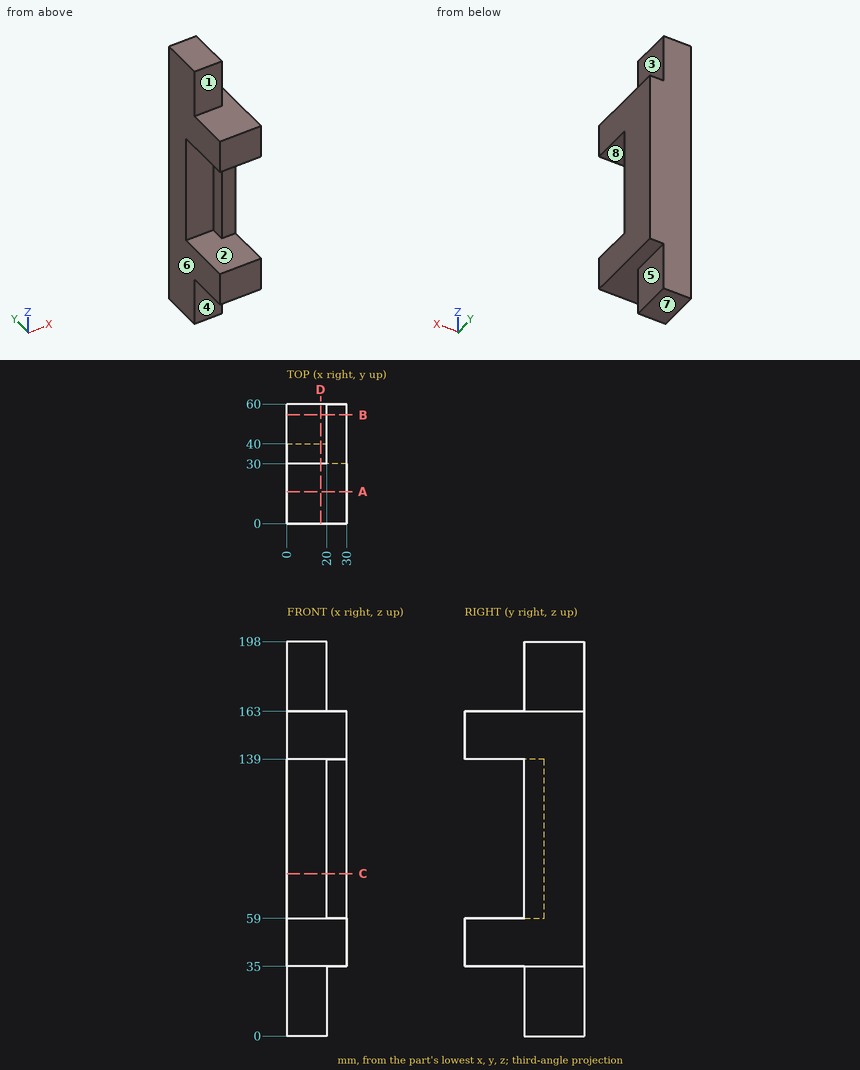
Can you work these out from the drawing? Everything is in mm from the part's minimum corner. A direction names the side the tool comes from. Give positions to 0.01 mm unless a question says otherwise; leave off trailing zeros. Write each loop counter-clockwise with the first axis right and the second up, starting at its lowest first coordinate (ties: lowest second). Pieces come first, ordered by that corner, then holes. Notation, with made-up numbers: M 40,3.5 L 46,3.5 A32 ccw 46,41.5 Z; hole C 76,-2 d2. An arc over 180 degrees is marked long. Answer in a Markdown table with one row per item. Add a question column.
Item 1: Imagine slicing it at D-D, the plane x = 17. Write out the boundary of the cut face in (y, z), plus the area to 3 significant figures.
Item 2: On a 3-axis mill with a long thin cutter (end or side, diameter ignored), from which of +Z, -Z, +X, -X, +Y, -Y can I reach the whole of each face in a straight line? I mean the marked faces 1, 2, 3, 4 and 5. Say none if no direction works.
Item 3: We'd pull the mould along Z, two halves only. Please class the marked faces 6, 7 and 8: released by +Z, released by -Z, zero draft, split by the parting line, or undercut.
Item 4: Imagine slicing it at A-A, the plane y = 16. Write out the boundary of the cut face in (x, z).
Item 5: Please list where these lines run through material, in increasing order: L1, parallel to Z at x = 11, y = 10.5; L2, parallel to Z at x = 4, y = 38; L3, parallel to Y at x = 25.25, z = 96.
Item 6: Imagine slicing it at C-C, the plane z = 81.5. Write out the boundary of the cut face in (x, y), plus the area to 3 significant figures.
Item 7: Imagine slicing it at B-B, the plane y = 54.5. Write out the boundary of the cut face in (x, z), plus the area to 3 significant figures.
Item 8: For pin 1 Ø6 at (x, z) = (13.5, 25) entering from -Y; pin 2 Ø15 at (x, y) = (10, 37.5) entering from -Z; pin 3 Ø10 at (x, y) = (6.5, 24) entering from +Z; pin 4 Ø24 at (y, z) = (43, 179) entering from +X, each with a flat end and sliding along its axis, tell me the tip position at first contact or that it passes through.
Evaluation:
| question | item | result |
|---|---|---|
| 1 | outline | M 0,35 L 30,35 L 30,0 L 60,0 L 60,198 L 30,198 L 30,163 L 0,163 L 0,139 L 40,139 L 40,59 L 0,59 Z |
| 1 | area | 6,580 mm² |
| 2 | face 1 | +Z, +X, -X, -Y |
| 2 | face 2 | -X, -Y |
| 2 | face 3 | +Z, +X, +Y, -Y |
| 2 | face 4 | -Z, +X, -X, -Y |
| 2 | face 5 | -Z, +X, +Y, -Y |
| 3 | face 6 | zero draft |
| 3 | face 7 | released by -Z |
| 3 | face 8 | undercut |
| 4 | outline | M 0,35 L 30,35 L 30,59 L 0,59 Z; M 0,139 L 30,139 L 30,163 L 0,163 Z |
| 5 | L1 | z = 35 to 59, 139 to 163 |
| 5 | L2 | z = 0 to 59, 139 to 198 |
| 5 | L3 | y = 30 to 60 |
| 6 | outline | M 0,40 L 20,40 L 20,30 L 30,30 L 30,60 L 0,60 Z |
| 6 | area | 700 mm² |
| 7 | outline | M 0,0 L 20,0 L 20,35 L 30,35 L 30,163 L 20,163 L 20,198 L 0,198 Z |
| 7 | area | 5,240 mm² |
| 8 | pin 1 | stops at y = 30 |
| 8 | pin 2 | stops at z = 0 |
| 8 | pin 3 | stops at z = 163 |
| 8 | pin 4 | stops at x = 20 |
